For this review, take the finished solid that the model builds, in its own axes (mm). A direction names the side the tool comes from. Coordinates: 2 decimals unless noted, no trailing zeros. Loops run counter-clockwise (first coordinate to the right, second up) from the corner with the lowest first, then second, coordinate; pieces in that order, holes last. Notation, with made-up numbers: M 71,-36.5 L 128,-36.5 A15 ccw 128,-23.5 Z; hole C 30,52 d2. An arc over 180 degrees is marked long. Put each result on its own line as item: value.
```python
from build123d import *

# Parameters (mm, degrees)
SKETCH_1_R             = 7
EXTRUDE_1_DEPTH        = 89
SKETCH_2_R             = 2
EXTRUDE_2_DEPTH        = 16
SKETCH_3_R             = 6
EXTRUDE_3_DEPTH        = 14
CHAMFER_1_SIZE         = 3
EXTRUDE_4_DEPTH        = 8
PATTERN_LINEAR_1_COUNT = 2
PATTERN_LINEAR_1_PITCH = 20


with BuildPart() as part:
    # 草图1 → 凸台-拉伸1 (new body)
    with BuildSketch(Plane.XY):
        Circle(SKETCH_1_R)
    extrude(amount=EXTRUDE_1_DEPTH)

    # 草图2 → 凸台-拉伸2 (add)
    with BuildSketch(Plane.XY.offset(89)):
        Circle(SKETCH_2_R)
    extrude(amount=EXTRUDE_2_DEPTH)

    # 草图3 → 凸台-拉伸3 (add)
    with BuildSketch(Plane.XY.offset(105)):
        Circle(SKETCH_3_R)
    extrude(amount=EXTRUDE_3_DEPTH)

    # 倒角1
    chamfer_1_edges = [part.edges().sort_by_distance(p)[0] for p in [
        (-6, 0, 119),
    ]]
    chamfer(chamfer_1_edges, length=CHAMFER_1_SIZE)

    # 草图4 → 凸台-拉伸4 (add)
    with BuildSketch(Plane(origin=(0, 0, 25), x_dir=(-1, 0, 0), z_dir=(0, 0, -1))):
        Polygon((-3.277805691, 10.468491925), (-10.704882792, 2.395582966), (-7.427077101, -8.07290896), (3.277805691, -10.468491925), (10.704882792, -2.395582966), (7.427077101, 8.07290896), align=None)
    extrude_4 = extrude(amount=EXTRUDE_4_DEPTH)

    # 阵列(线性)1: 凸台-拉伸4 ×2
    with Locations(*[(0, 0, i * PATTERN_LINEAR_1_PITCH) for i in range(1, PATTERN_LINEAR_1_COUNT)]):
        add(extrude_4)


solid = part.part
```
(1) Draft analysis for pull direction Z (two halves, no side actions). For faces 1 (the cylindrical face through (-6, 0, 110)), 2 (the cylindrical face through (6.466, -2.681, 30.916)), 3 (the cylindrical face through (0, -2, 97)), 4 (the flat face through (0, 0, 119)), state which applies: +Z half, -Z half, draft (parallel to the pull), parting line (faces both ways), or undercut.
Determined:
face 1: draft
face 2: undercut
face 3: undercut
face 4: +Z half
(2) Add section B-B (x = 9.25). Write out the cut boundary in (y, z), plus the area to 3 significant figures.
Determined:
outline: M -2.25,17 L 3.98,17 L 3.98,25 L -2.25,25 Z; M -2.25,37 L 3.98,37 L 3.98,45 L -2.25,45 Z
area: 99.6 mm^2
(3) Tool access review of faces 5 (the flat face through (6.4, 3.2, 25)), 6 (the flat face through (6.4, 3.2, 17)), 7 (the flat face through (6.4, 3.2, 45)): name each direction out of +Z, -Z, +X, -X, +Y, -Y from which nothing blocks a thin tool from reaching the whole face with its end or side.
Determined:
face 5: none
face 6: -Z
face 7: +Z
(4) Wall thickness on line 1 along Z through (x, y) = (-8.75, 1.5); line 2 along X through (y, z) = (0, 62.5); line 3 along Z through (x, y) = (4.75, 1): over which ranges is each line inside the solid? List them lowest first. Write a range as [from, to].
Determined:
line 1: z = [17, 25], [37, 45]
line 2: x = [-7, 7]
line 3: z = [0, 89], [105, 117.15]
(5) For pin 1 (6 mm diameter, centred on x = 7, z = 24, fed in from +Y); pin 2 (2 mm diameter, centred on y = 7, z = 22.5, fed in from -X); pin 3 (4 mm diameter, centred on y = -7.5, z = 61.5, fed in from +X), all flat-tipped, find the tip position at first contact; note any pin that passes through.
Determined:
pin 1: stops at y = 9.68
pin 2: stops at x = -8.08
pin 3: stops at x = 4.33
(6) Add section D-D (z = 60). Write out the cut boundary in (x, y).
Determined:
outline: C 0,0 d14
